Here's how the part is built. I have some questions about the finished solid (model axes, mm). A direction names the side the tool comes from. Coordinates: 2 decimals unless noted, no trailing zeros. Loops run counter-clockwise (first coordinate to the right, second up) from the corner with the lowest first, then second, coordinate; pieces in that order, holes last. Notation, with made-up numbers: M 55,42.5 L 60,42.5 A25 cw 60,79.5 Z; hole C 88.5,42.25 d2. An arc over 180 degrees is marked long. Use CSV: the item, a comma, the result in double quotes. Start each with the question number.
Q1. Please list where these lines run through material, in increasing order: probe 1 along Y at (x, z) = (-5.75, 9.75); probe 2 along X at (y, z) = (-3.25, 12.75); probe 3 along Y at (x, z) = (-11.75, 9.25). Write a range as [from, to].
Q2. If we section it at B-B (y = -8.5): Please give me the cut outline in (x, z), and give its area (3 significant figures).
Q3. If we mould it in two halves opening along X, with no side actions, what happens to faces 1 (the flat face through (-14.589, -3, 10)), 2 (the flat face through (-12, -0.5, 9.6)), 3 (the flat face through (-1, -4, 10)), 4 (the flat face through (-13, -10, 10))? For each: +X half, -X half, draft (parallel to the pull), parting line (faces both ways), or undercut.
Q4. For pin 1 Ø1.2 at (x, z) = (-9.5, 13) entering from +Y; pin 2 Ø1.2 at (x, z) = (-9.5, 10) entering from -Y, each with a flat end and sliding along its axis, tell me the tip position at first contact or that it passes through.
Q5. Which directions (+Z, -Z, +X, -X, +Y, -Y) give clear straight access to the entire face, cutting with the end or side of a thin tool? Please do faces 5 (the flat face through (-4, -7, 16)), 6 (the flat face through (-10, -11, 10)), 7 (the flat face through (-13, -7, 10)), 8 (the flat face through (-13, -17, 10)).
Q6. If we section it at D-D (y = -6.5): Please give me the cut outline in (x, z).
Q7. If we section it at A-A (x = -5): Please give me the cut outline in (y, z), and give its area (3 significant figures).
Q8. If we section it at C-C (x = -10.5): Please give me the cut outline in (y, z).
from build123d import *

# Parameters (mm, degrees)
CROQUIS2_W              = 6
CROQUIS2_H              = 5
SALIENTE_EXTRUIR1_DEPTH = 19.5
CORTAR_EXTRUIR1_REACH   = 29.079
CROQUIS4_R              = 1.5
CROQUIS4_W              = 7
CROQUIS4_H              = 3


with BuildPart() as part:
    # Croquis2 → Saliente-Extruir1 (new body)
    # profile 1 of 2: a face of its own
    with BuildSketch(Plane.XY):
        Polygon((0, -7), (0, 0), (-8, 0), (-8, -1), (-12, -1), (-12, 0), (-14.589269471, 0), (-14.589269471, -7), (-12, -7), (-12, -6), (-8, -6), (-8, -7), (-8, -8.5), (0, -8.5), align=None)
        Polygon((-8, -2), (-8, -3.5), (-8, -5), (-12, -5), (-12, -2), align=None, mode=Mode.SUBTRACT)
        with Locations((-4, -3.5)):
            Rectangle(CROQUIS2_W, CROQUIS2_H, mode=Mode.SUBTRACT)
    # profile 2 of 2: a face of its own
    with BuildSketch(Plane.XY):
        Polygon((0, -10), (0, -8.5), (-8, -8.5), (-8, -10), (-8, -11), (-12, -11), (-12, -10), (-14.589269471, -10), (-14.589269471, -17), (-12, -17), (-12, -16), (-8, -16), (-8, -17), (0, -17), align=None)
        Polygon((-12, -12), (-8, -12), (-8, -13.5), (-8, -15), (-12, -15), align=None, mode=Mode.SUBTRACT)
        with Locations((-4, -13.5)):
            Rectangle(CROQUIS2_W, CROQUIS2_H, mode=Mode.SUBTRACT)
    extrude(amount=SALIENTE_EXTRUIR1_DEPTH)

    # Croquis4 → Cortar-Extruir1 (cut, up to next)
    with BuildSketch(Plane.ZY.offset(8), mode=Mode.PRIVATE) as cortar_extruir1_sk1:
        with Locations((9.75, -8.5)):
            Circle(CROQUIS4_R)
    cortar_extruir1_tool1 = extrude(cortar_extruir1_sk1.sketch, amount=-CORTAR_EXTRUIR1_REACH, mode=Mode.PRIVATE) & part.part
    # Croquis4 → Cortar-Extruir1 (cut, up to next)
    with BuildSketch(Plane.ZY.offset(8), mode=Mode.PRIVATE) as cortar_extruir1_sk2:
        with Locations((3.5, -8.5)):
            Rectangle(CROQUIS4_W, CROQUIS4_H)
    cortar_extruir1_tool2 = extrude(cortar_extruir1_sk2.sketch, amount=-CORTAR_EXTRUIR1_REACH, mode=Mode.PRIVATE) & part.part
    # Croquis4 → Cortar-Extruir1 (cut, up to next)
    with BuildSketch(Plane.ZY.offset(8), mode=Mode.PRIVATE) as cortar_extruir1_sk3:
        with Locations((16, -8.5)):
            Rectangle(CROQUIS4_W, CROQUIS4_H)
    cortar_extruir1_tool3 = extrude(cortar_extruir1_sk3.sketch, amount=-CORTAR_EXTRUIR1_REACH, mode=Mode.PRIVATE) & part.part
    add(cortar_extruir1_tool1.solids().sort_by_distance((-8, -8.5, 9.75))[0], mode=Mode.SUBTRACT)
    add(cortar_extruir1_tool2.solids().sort_by_distance((-8, -8.5, 3.5))[0], mode=Mode.SUBTRACT)
    add(cortar_extruir1_tool3.solids().sort_by_distance((-8, -8.5, 16))[0], mode=Mode.SUBTRACT)


solid = part.part
Results below:
1,probe 1,"[-17, -16], [-11, -10], [-7, -6], [-1, 0]"
1,probe 2,"[-14.59, -12], [-8, -7], [-1, 0]"
1,probe 3,"[-16, -15], [-12, -11], [-6, -5], [-2, -1]"
2,outline,"M -8,7 L 0,7 L 0,8.25 L -8,8.25 Z; M -8,11.25 L 0,11.25 L 0,12.5 L -8,12.5 Z"
2,area,"20.0 mm^2"
3,face 1,"-X half"
3,face 2,"undercut"
3,face 3,"undercut"
3,face 4,"draft"
4,pin 1,"y = -1"
4,pin 2,"y = -16"
5,face 5,"+Z, +X, -X"
5,face 6,"+Z, -Z"
5,face 7,"+Z, -Z, -X"
5,face 8,"+Z, -Z, +X, -X, -Y"
6,outline,"M -14.59,0 L -12,0 L -12,19.5 L -14.59,19.5 Z; M -8,0 L 0,0 L 0,19.5 L -8,19.5 Z"
7,outline,"M -17,0 L -16,0 L -16,19.5 L -17,19.5 Z; M -11,0 L -10,0 L -10,7 L -7,7 L -7,0 L -6,0 L -6,19.5 L -7,19.5 L -7,12.5 L -10,12.5 L -10,19.5 L -11,19.5 Z; M -1,0 L 0,0 L 0,19.5 L -1,19.5 Z; hole C -8.5,9.75 d3"
7,area,"87.4 mm^2"
8,outline,"M -16,0 L -15,0 L -15,19.5 L -16,19.5 Z; M -12,0 L -11,0 L -11,19.5 L -12,19.5 Z; M -6,0 L -5,0 L -5,19.5 L -6,19.5 Z; M -2,0 L -1,0 L -1,19.5 L -2,19.5 Z"
